Part print with two shaded views. Sizes in mm from the minimum x, y, z corner. Round coordinates to 2 decimals unless told otherwise and drop trailing zeros. Write each loop counter-clockwise with the first axis right and the second up, starting at its lowest first coordinate (ties: lowest second). Pieces come first, ordered by that corner, then holes.
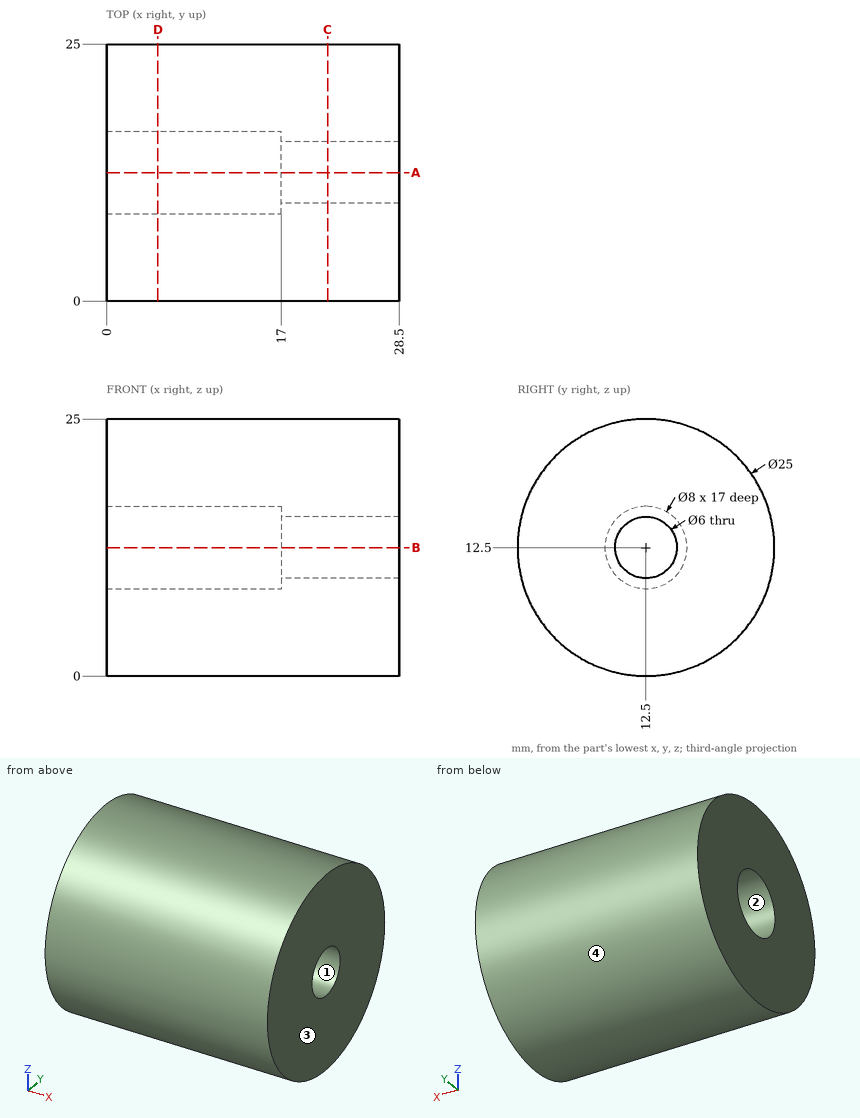
Q1. Mould opens along Z. For the marked faces 1, 2, 3 and 4 say: +Z half, -Z half, draft (parallel to the pull), parting line (faces both ways), or undercut.
Values follow:
face 1: undercut
face 2: undercut
face 3: draft
face 4: parting line
Q2. Drop flat-ended pins along their axis: pin 1 (1.5 mm diameter, centred on x = 13, y = 8.5, fed in from +Z); pin 2 (2 mm diameter, centred on x = 13.5, y = 15.5, fed in from -Z); pin 3 (2 mm diameter, centred on x = 16, y = 20, fed in from +Z). Give the stop position or say it passes through.
Values follow:
pin 1: stops at z = 24.57
pin 2: stops at z = 0.16
pin 3: stops at z = 23.18
Q3. Cut at D-D on x = 5. Write the cut outline in (y, z), plus the area to 3 significant figures.
Values follow:
outline: circle Ø25 at (12.5, 12.5); hole circle Ø8 at (12.5, 12.5)
area: 441 mm2
Q4. Cut at C-C on x = 21.5. Write the cut outline in (y, z).
Values follow:
outline: circle Ø25 at (12.5, 12.5); hole circle Ø6 at (12.5, 12.5)
Q5. Wall check: L1, parallel to Z at x = 20.5, y = 12.5; L2, parallel to Z at x = 7.25, y = 12.5; L3, parallel to Y at x = 5.25, z = 14.75. Give the ranges that are in metal, low to high.
Values follow:
L1: z = 0 to 9.5, 15.5 to 25
L2: z = 0 to 8.5, 16.5 to 25
L3: y = 0.2 to 9.19, 15.81 to 24.8
Q6. Cut at A-A on y = 12.5. Write the cut outline in (x, z), plus the area to 4 significant figures.
Values follow:
outline: (0, 0) - (28.5, 0) - (28.5, 9.5) - (17, 9.5) - (17, 8.5) - (0, 8.5) - close; (0, 16.5) - (17, 16.5) - (17, 15.5) - (28.5, 15.5) - (28.5, 25) - (0, 25) - close
area: 507.5 mm2
